Part model, mm, in its own coordinate system. Face numbers are marked on the shaded views. A direction names the side the tool comes from. Coordinates: 2 decimals unless noted, no trailing zeros. Order: outer loops, then holes, each group sorted by start corner. A loop starts at its lowest first (then second) coordinate and runs counter-clockwise, first axis right, second up.
1) Cut at B-B (z = 0.5). List the corners of the cut face in (x, y) (3 decimals).
2) Cut at A-A (x = 0). List the corners of the cut face in (y, z) (3 decimals), and give its area (3 significant figures).
3) Pin check, flat tips, straight feed: pin 1 Ø3 at (y, z) = (-4.5, 6.5) entering from +X; pin 2 Ø1 at (x, z) = (10.5, 3.5) entering from +Y; pin 3 Ø10 at (x, y) = (8.5, -4.5) entering from -Z; pin 4 Ø3 at (y, z) = (-3, 4.5) entering from -X. Stop position of each tip, or through.
4) Cut at D-D (z = 4.5). Give the number of separate pieces and of enclosed holes in the cut face, and give its area (3 significant figures).
5) Mould opens along X. For the marked faces 1 and 2 say: +X half, -X half, draft (parallel to the pull), parting line (faces both ways), or undercut.
6) Wall check: L1, parallel to Y at x = 0, z = 2.7 (3 decimals); L2, parallel to Z at x = 2.5, y = 10; L3, parallel to Y at x = -4, z = 5.5. Give the ranges that are in metal, low to high.
7) Cut at C-C (y = 5). List the corners of the cut face in (x, z).
8) Tool access for the marked faces 3 and 4: list every direction of +Z, -Z, +X, -X, +Y, -Y with a clear straight run to the whole face (end or side of a thin tool).
```python
from build123d import *

# Parameters (mm, degrees)
F1_DEPTH = 3.81
F3_DEPTH = 3.556
F4_R     = 0.254
F6_COUNT = 6
F8_R     = 9.525
F9_DEPTH = 3.81


with BuildPart() as f1:
    # F0 (on Top) → F1 (new body)
    with BuildSketch(Plane.XY):
        Polygon((6.4951905284, 11.25), (-6.4951905284, 11.25), (-12.9903810568, 0), (-6.4951905284, -11.25), (6.4951905284, -11.25), (12.9903810568, 0), align=None)
    extrude(amount=F1_DEPTH)

    # F2 (on face) → F3 (join)
    with BuildSketch(Plane.XY.offset(3.81)):
        with BuildLine():
            Line((12.9903810568, 0), (9.7427857926, 5.625))
            ThreePointArc((9.7427857926, 5.625), (11.25, 0), (9.7427857926, -5.625))
            Line((9.7427857926, -5.625), (12.9903810568, 0))
        make_face()
    extrude(amount=F3_DEPTH)

    # F4
    f4_edges = [f1.edges().sort_by_distance(p)[0] for p in [
        (9.742786, -5.625, 5.588),
        (9.742786, 5.625, 5.588),
    ]]
    fillet(f4_edges, radius=F4_R)

    # F6: F1 ×6 about axis
    f6_axis = Axis((0, 0, 19.5707920939), (0, 0, 1))


with BuildPart() as f1_1:
    add(f1.part)
    for i in range(1, F6_COUNT):
        add(f1.part.rotate(f6_axis, i * 360 / F6_COUNT))

    # F8 (on face) → F9 (cut, through all)
    with BuildSketch(Plane.XY.offset(3.81)):
        Circle(F8_R)
    extrude(amount=-F9_DEPTH, mode=Mode.SUBTRACT)


solid = f1_1.part
```
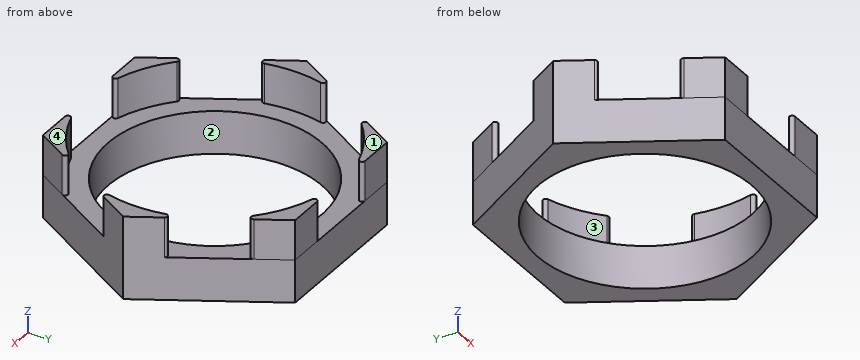
Geometry check:
1. outline: (-12.99, 0) - (-6.495, -11.25) - (6.495, -11.25) - (12.99, 0) - (6.495, 11.25) - (-6.495, 11.25) - close; hole circle Ø19.05 at (0, 0)
2. outline: (-11.25, 0) - (-9.525, 0) - (-9.525, 3.81) - (-11.25, 3.81) - close; (9.525, 0) - (11.25, 0) - (11.25, 3.81) - (9.525, 3.81) - close
2. area: 13.1 mm2
3. pin 1: passes through
3. pin 2: stops at y = 5.18
3. pin 3: stops at z = 0
3. pin 4: stops at x = -12.12
4. separate pieces: 6
4. enclosed holes: 0
4. area: 35.1 mm2
5. face 1: draft
5. face 2: undercut
6. L1: y = -11.25 to -9.525, 9.525 to 11.25
6. L2: z = 0 to 3.81
6. L3: y = -11.25 to -10.51, 10.51 to 11.25
7. outline: (-10.1, 0) - (-8.11, 0) - (-8.11, 3.81) - (-10.1, 3.81) - close; (8.11, 0) - (10.1, 0) - (10.1, 3.81) - (8.11, 3.81) - close
8. face 3: +Z
8. face 4: +Z, +X, -X, +Y, -Y
